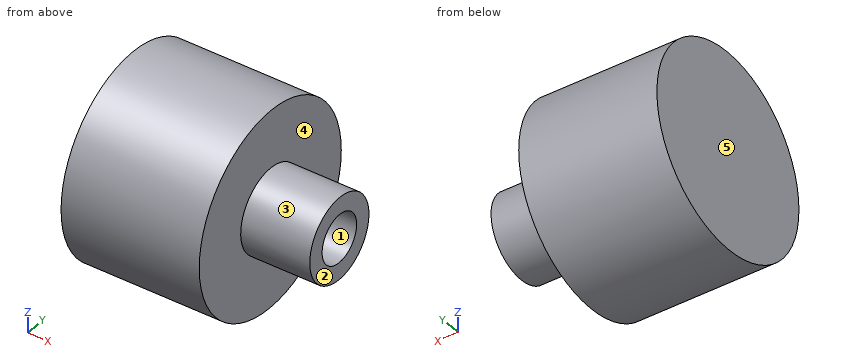
Autodesk Inventor part; units mm, degrees
ref_plane "YZ Plane" through (0, 0, 0) normal (1, 0, 0) x (0, 1, 0)
ref_plane "XZ Plane" through (0, 0, 0) normal (0, 1, 0) x (-1, 0, 0)
ref_plane "XY Plane" through (0, 0, 0) normal (0, 0, 1) x (1, 0, 0)
sketch "Sketch1" plane through (0, 0, 0) normal (1, 0, 0) x (0, 1, 0)
  circle A0 centre (0, 0) radius 14.4
  dimension "d0" = 28.8
extrude "Extrusion1" add sketch "Sketch1" along normal blind 20
sketch "Sketch2" plane through (20, 0, 0) normal (1, 0, 0) x (0, 0, -1)
  circle A0 centre (0, 0) radius 3.5
  circle A1 centre (0, 0) radius 6
  dimension "d3" = 7
  dimension "d4" = 12
extrude "Extrusion2" add sketch "Sketch2" along normal blind 10 contours A0 | A1
sketch "Sketch3" plane through (30, 0, 0) normal (1, 0, 0) x (0, 0, -1)
  circle A0 centre (0, 0) radius 3.5
  dimension "d7" = 7
extrude "Extrusion3" cut sketch "Sketch3" against normal blind 25
properties part number "wheels" material "Rubber"
Can you work these out from the model? Positions are in its coordinate system, mm. Face numbers are marked on the shaded views. A direction names the side the tool comes from. Give positions to 0.01 mm unless a question says otherwise; leave off trailing zeros. Loops run counter-clockwise (first coordinate to the right, second up) from the corner with the lowest first, then second, coordinate; pieces in that order, holes last. Notation, with made-up numbers: (15, -27) -> (33, -27) arc R22 ccw to (33, -20) -> close; hole circle Ø9 at (-27, 45). An arc over 180 degrees is marked (long way). Write item = value, one per line.
1) Thinking about a two-plate mould opening in Y: for the marked faces 1, 2 and 3, which applies, released by +Y, released by -Y, zero draft, split by the parting line, or undercut?
Check result:
face_1 = undercut
face_2 = zero draft
face_3 = split by the parting line
2) Suppose I cut it at D-D on z = 4.5. Write out the boundary of the cut face in (x, y), then the cut area to 3 significant figures.
Check result:
outline = (0, -13.68) -> (20, -13.68) -> (20, -3.97) -> (30, -3.97) -> (30, 3.97) -> (20, 3.97) -> (20, 13.68) -> (0, 13.68) -> close
area = 627 mm2
3) I need wall thicknesses on L1, parallel to X at y = 6.5, z = -9.5; L2, parallel to X at y = -0.5, z = 1; L3, parallel to Y at x = 12.75, z = 2. Which ranges of each line are inside material? Lowest first, please. Write a range as from..to.
Check result:
L1 = 0..20
L2 = 0..5
L3 = -14.26..-2.87, 2.87..14.26
4) Will these pins go through, and if not, where does the flat tip stop? pin 1 (5 mm diameter, centred on x = 3, y = -3, fed in from +Z); pin 2 (4 mm diameter, centred on y = 1, z = 11.5, fed in from -X); pin 3 (3 mm diameter, centred on y = -9.5, z = -2, fed in from +X); pin 4 (1.5 mm diameter, centred on x = 10.5, z = -7, fed in from -Y).
Check result:
pin_1 = 14.39
pin_2 = 0
pin_3 = 20
pin_4 = -12.97
5) For the marked faces 4 and 5, which set-ups out of +Z, -Z, +X, -X, +Y, -Y let a thin tool reach every point of the face, with its end or its side?
Check result:
face_4 = +X
face_5 = +Z, -Z, -X, +Y, -Y
6) Suppose I cut it at C-C on x = 27.5. Write out the boundary of the cut face in (y, z).
Check result:
outline = circle Ø12 at (0, 0); hole circle Ø7 at (0, 0)
7) Suppose I cut it at A-A on y = 0. Write out the boundary of the cut face in (x, z), then the cut area to 3 significant figures.
Check result:
outline = (0, -14.4) -> (20, -14.4) -> (20, -6) -> (30, -6) -> (30, -3.5) -> (5, -3.5) -> (5, 3.5) -> (30, 3.5) -> (30, 6) -> (20, 6) -> (20, 14.4) -> (0, 14.4) -> close
area = 521 mm2
